```python
from build123d import *

# Parameters (mm, degrees)
F1_DEPTH       = 20
F2_R           = 3.075
F3_DEPTH       = 1.7
F5_DEPTH       = 5
F6_W           = 5
F6_H           = 8.5
F7_DEPTH       = 1.4
F10_DEPTH      = 1
F12_DEPTH      = 2.3
F13_R          = 1
F14_DEPTH      = 9.4
F14_DEPTH_BACK = 28.6
F15_R          = 1.2
F16_SIZE       = 0.2
F18_DEPTH      = 5


with BuildPart() as f1:
    # F0 (on Right) → F1 (new body)
    with BuildSketch(Plane.YZ):
        with BuildLine():
            Line((6.6332495807, 7.55), (-6.6332495807, 7.55))
            ThreePointArc((-6.6332495807, 7.55), (-10.05, 0), (-6.6332495807, -7.55))
            Line((-6.6332495807, -7.55), (6.6332495807, -7.55))
            ThreePointArc((6.6332495807, -7.55), (10.05, 0), (6.6332495807, 7.55))
        make_face()
    extrude(amount=F1_DEPTH)

    # F2 (on face) → F3 (join)
    with BuildSketch(Plane.YZ.offset(20)):
        Circle(F2_R)
    extrude(amount=F3_DEPTH)

    # F4 (on face) → F5 (join)
    with BuildSketch(Plane(origin=(0, 0, 0), x_dir=(0, -1, 0), z_dir=(-1, 0, 0))):
        with BuildLine():
            Line((6.6143782777, 7.5), (-6.6143782777, 7.5))
            ThreePointArc((-6.6143782777, 7.5), (-10, 0), (-6.6143782777, -7.5))
            Line((-6.6143782777, -7.5), (6.6143782777, -7.5))
            ThreePointArc((6.6143782777, -7.5), (10, 0), (6.6143782777, 7.5))
        make_face()
    extrude(amount=F5_DEPTH)

    # F6 (on face) → F7 (join)
    with BuildSketch(Plane.XY.offset(7.5)):
        with Locations((-2.5, 0)):
            Rectangle(F6_W, F6_H)
    extrude(amount=F7_DEPTH)

    # F9 (on offset) → F10 (join, symmetric)
    with BuildSketch(Plane(origin=(-1.6, 0, 0), x_dir=(0, -1, 0), z_dir=(-1, 0, 0))):
        Polygon((4.25, 7.6051868729), (4.25, 7.5), (8.25, 8.8049311029), (8.2189854098, 8.9), align=None)
        Polygon((-8.25, 8.8049311029), (-4.25, 7.5), (-4.25, 7.6051868729), (-8.2189854098, 8.9), align=None)
    extrude(amount=F10_DEPTH, both=True)

    # F11 (on face) → F12 (join)
    with BuildSketch(Plane(origin=(-5, 0, 0), x_dir=(0, -1, 0), z_dir=(-1, 0, 0))):
        with BuildLine():
            Line((-3.5707142143, -3.5), (3.5707142143, -3.5))
            ThreePointArc((3.5707142143, -3.5), (0, 5), (-3.5707142143, -3.5))
        make_face()
    extrude(amount=F12_DEPTH)

    # F13 (on face) → F14 (join, two sides)
    with BuildSketch(Plane.YZ.offset(20)) as f14_sk:
        Circle(F13_R)
    extrude(amount=F14_DEPTH)
    extrude(f14_sk.sketch, amount=-F14_DEPTH_BACK)

    # F15
    f15_edges = [f1.edges().sort_by_distance(p)[0] for p in [
        (-5, -10, 0),
        (-5, 10, 0),
        (-5, 0, 8.9),
        (20, -10.05, 0),
        (20, 10.05, 0),
    ]]
    fillet(f15_edges, radius=F15_R)

    # F16
    f16_edges = [f1.edges().sort_by_distance(p)[0] for p in [
        (-8.6, -1, 0),
        (-7.3, 0, 5),
        (21.7, -3.075, 0),
        (29.4, -1, 0),
        (-7.3, 0, -3.5),
    ]]
    chamfer(f16_edges, length=F16_SIZE)

    # F17 (on face) → F18 (cut)
    with BuildSketch(Plane(origin=(-5, 0, 0), x_dir=(0, -1, 0), z_dir=(-1, 0, 0))):
        with BuildLine():
            Line((12, 1.25), (10, 1.25))
            ThreePointArc((10, 1.25), (8.75, 0), (10, -1.25))
            Line((10, -1.25), (12, -1.25))
            Line((12, -1.25), (12, 1.25))
        make_face()
        with BuildLine():
            Line((-12, -1.25), (-10, -1.25))
            ThreePointArc((-10, -1.25), (-8.75, 0), (-10, 1.25))
            Line((-10, 1.25), (-12, 1.25))
            Line((-12, 1.25), (-12, -1.25))
        make_face()
    extrude(amount=-F18_DEPTH, mode=Mode.SUBTRACT)


solid = f1.part
```
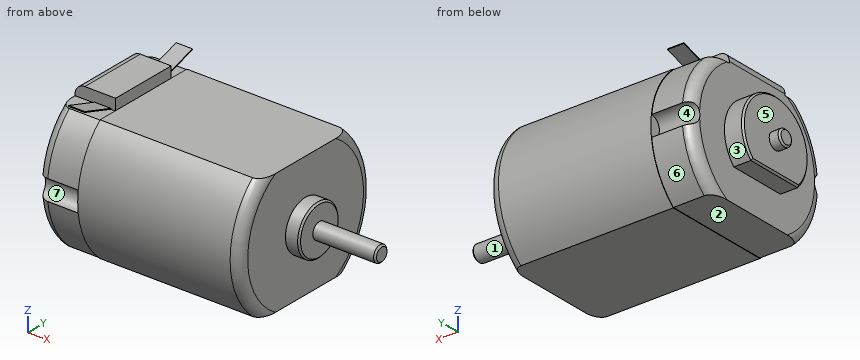
Geometry: final body of the model. Coordinates: model frame, mm. Face numbers are marked on the shaded views. A direction names the side the tool comes from. Round coordinates to 2 decimals unless told otherwise and drop trailing zeros. Loops run counter-clockwise (first coordinate to the right, second up) from the corner with the lowest first, then second, coordinate; pieces in that order, holes last. Notation, with made-up numbers: (85, 80) -> (120, 80) arc R20 ccw to (120, 104) -> close; hole circle Ø1 at (10.5, 35). An arc over 180 degrees is marked (long way). Use one line per item in the form item = value.
Item 1: Cut plane A-A on x = -1. Output: boundary loops of the cut face in (y, z).
Evaluation:
outline = (-9.92, -1.25) arc R10 ccw to (-6.61, -7.5) -> (6.61, -7.5) arc R10 ccw to (9.92, -1.25) arc R1.25 cw to (9.92, 1.25) arc R10 ccw to (6.61, 7.5) -> (4.25, 7.5) -> (8.25, 8.8) -> (8.22, 8.9) -> (4.25, 7.61) -> (4.25, 8.9) -> (-4.25, 8.9) -> (-4.25, 7.61) -> (-8.22, 8.9) -> (-8.25, 8.8) -> (-4.25, 7.5) -> (-6.61, 7.5) arc R10 ccw to (-9.92, 1.25) arc R1.25 cw to start
Item 2: Cut plane C-C on x = 3. Output: boundary loops of the cut face in (y, z), then the cut area to 3 significant figures.
Evaluation:
outline = (-6.63, -7.55) -> (6.63, -7.55) arc R10.05 ccw to (6.63, 7.55) -> (-6.63, 7.55) arc R10.05 ccw to start
area = 272 mm2
Item 3: Material intervals for probe 1 along X at (y, z) = (-2.5, 0.5); probe 2 along Z at (x, y) = (15, 0.75); probe 3 along Z at (x, y) = (-2, -3.75), sorted ascending.
Evaluation:
probe_1 = -7.3 to 21.7
probe_2 = -7.55 to 7.55
probe_3 = -7.5 to 8.9
Item 4: Draft query along Z for the marked faces 4, 5, 6 and 7. Return one class per face: released by +Z, released by -Z, zero draft, split by the parting line, or undercut.
Evaluation:
face_4 = undercut
face_5 = zero draft
face_6 = released by -Z
face_7 = undercut
Item 5: Access query for the marked faces 1, 2 and 3. Directions: +Z, -Z, +X, -X, +Y, -Y. A direction counts if a zero-diameter tool reaches every point of the face in a straight line with its end or side. Return the directions, or none.
Evaluation:
face_1 = +X
face_2 = -Z, -X, +Y, -Y
face_3 = -X
Item 6: Cut plane D-D on x = 20.5. Output: boundary loops of the cut face in (y, z) (3 decimals).
Evaluation:
outline = circle Ø6.15 at (0, 0)
Item 7: Contact query for flat-ended pins moving along their axis: pin 1 Ø2.5 at (x, y) = (-2, 6) entering from +Z; pin 2 Ø1.5 at (y, z) = (2.5, 5) entering from +X; pin 3 Ø8 at (y, z) = (4.5, 0) entering from +X; pin 4 Ø1 at (x, z) = (23, 1) entering from -Y. Output: stop coordinate, or through.
Evaluation:
pin_1 = 8.58
pin_2 = 20
pin_3 = 29.4
pin_4 = -0.87
